```python
from build123d import *

# Parameters (mm, degrees)
BOSS_EXTRUDE1_DEPTH = 3
CUT_EXTRUDE1_DEPTH  = 3
FILLET1_R           = 5
CUT_EXTRUDE2_DEPTH  = 128.710610366


with BuildPart() as part:
    # Sketch1 → Boss-Extrude1 (new body)
    with BuildSketch(Plane(origin=(0, 0, 0), x_dir=(1, 0, 0), z_dir=(0, 1, 0))):
        Polygon((0, 0), (75, 0), (75, 15), (125, 15), (125, -26), (0, -26), align=None)
    extrude(amount=BOSS_EXTRUDE1_DEPTH)

    # Sketch2 → Cut-Extrude1 (cut)
    with BuildSketch(Plane(origin=(0, 3, 0), x_dir=(1, 0, 0), z_dir=(0, 1, 0))):
        with BuildLine():
            Line((92.84, 7), (92.84, -18))
            ThreePointArc((92.84, -18), (91.34, -19.5), (89.84, -18))
            Line((89.84, -18), (89.84, 7))
            ThreePointArc((89.84, 7), (91.34, 8.5), (92.84, 7))
        make_face()
        with BuildLine():
            Line((107.16, 7), (107.16, -18))
            ThreePointArc((107.16, -18), (108.66, -19.5), (110.16, -18))
            Line((110.16, -18), (110.16, 7))
            ThreePointArc((110.16, 7), (108.66, 8.5), (107.16, 7))
        make_face()
    extrude(amount=-CUT_EXTRUDE1_DEPTH, mode=Mode.SUBTRACT)

    # Fillet1
    fillet1_edges = [part.edges().sort_by_distance(p)[0] for p in [
        (75, 1.5, 0),
        (75, 1.5, -15),
        (125, 1.5, -15),
        (125, 1.5, 26),
    ]]
    fillet(fillet1_edges, radius=FILLET1_R)

    # Sketch4 → Cut-Extrude2 (cut, through all)
    with BuildSketch(Plane(origin=(0, 3, 0), x_dir=(1, 0, 0), z_dir=(0, 1, 0))):
        with BuildLine():
            Line((45, -21.5), (5, -21.5))
            ThreePointArc((5, -21.5), (3.5, -20), (5, -18.5))
            Line((5, -18.5), (45, -18.5))
            ThreePointArc((45, -18.5), (46.5, -20), (45, -21.5))
        make_face()
        with BuildLine():
            Line((45, -4.5), (5, -4.5))
            ThreePointArc((5, -4.5), (3.5, -6), (5, -7.5))
            Line((5, -7.5), (45, -7.5))
            ThreePointArc((45, -7.5), (46.5, -6), (45, -4.5))
        make_face()
    extrude(amount=-CUT_EXTRUDE2_DEPTH, mode=Mode.SUBTRACT)


solid = part.part
```
Verification items for the finished model (mm, model axes). A direction names the side the tool comes from. Coordinates: 2 decimals unless noted, no trailing zeros. Write each loop counter-clockwise with the first axis right and the second up, starting at its lowest first coordinate (ties: lowest second). Pieces come first, ordered by that corner, then holes. Notation, with made-up numbers: (-27.75, 21.5) - (15.25, 21.5) arc R22 cw to (15.25, 54.5) - close; hole circle Ø11 at (-28.5, -31.5). An arc over 180 degrees is marked (long way). One line per question, with ' | ' between items. Start each with the question number.
1. Section check A-A (z = 13). Enter the section's corners in (x, y), plus the area to 3 significant figures.
2. Gauge pin test, flat end, axial feed: P1, Ø1.5, axis at x = 23, y = 1.5, coming from the -Z side. Record the tip position at first contact, or that the pin passes through.
3. Draft check along Z on faces 1 (the cylindrical face through (123, 2, -14)), 2 (the flat face through (77, 0, 10)), 3 (the flat face through (25, 2, 7.5)), 4 (the flat face through (61, 1, 26)). Enter one of: released by +Z, released by -Z, zero draft, split by the parting line, or undercut.
4. Access from +Z, -Z, +X, -X, +Y, -Y to the whole of each face (thin tool, end or side, straight path). Record for faces 5 (the flat face through (100, 1, -15)), 6 (the flat face through (75, 1, -7)), 7 (the flat face through (25, 2, 18.5)).
5. Section check D-D (z = -11.5). Enter the section's corners in (x, y), plus the area to 3 significant figures.
6. Material ranges on line 1 along X through (y, z) = (1.2, 17); line 2 along Z through (x, y) = (18.5, 0.75); line 3 along X through (y, z) = (0.35, -9), recorded low to high.
7. Section check C-C (z = 6). Enter the section's corners in (x, y), plus the area to 3 significant figures.
8. Section check B-B (x = 108.66). Enter the section's corners in (y, z).
Computed values:
1) outline: (0, 0) - (89.84, 0) - (89.84, 3) - (0, 3) - close; (92.84, 0) - (107.16, 0) - (107.16, 3) - (92.84, 3) - close; (110.16, 0) - (125, 0) - (125, 3) - (110.16, 3) - close | area: 357 mm²
2) P1: z = 0
3) face 1: released by -Z | face 2: zero draft | face 3: undercut | face 4: released by +Z
4) face 5: -Z, +X, -X, +Y, -Y | face 6: -Z, -X, +Y, -Y | face 7: +Y, -Y
5) outline: (75.23, 0) - (124.77, 0) - (124.77, 3) - (75.23, 3) - close | area: 149 mm²
6) line 1: 0 to 89.84, 92.84 to 107.16, 110.16 to 125 | line 2: 0 to 4.5, 7.5 to 18.5, 21.5 to 26 | line 3: 75 to 125
7) outline: (0, 0) - (3.5, 0) - (3.5, 3) - (0, 3) - close; (46.5, 0) - (89.84, 0) - (89.84, 3) - (46.5, 3) - close; (92.84, 0) - (107.16, 0) - (107.16, 3) - (92.84, 3) - close; (110.16, 0) - (125, 0) - (125, 3) - (110.16, 3) - close | area: 228 mm²
8) outline: (0, -15) - (3, -15) - (3, -8.5) - (0, -8.5) - close; (0, 19.5) - (3, 19.5) - (3, 26) - (0, 26) - close
